Source: CAD feature listing. Evaluate the final solid. Frame: model axes, mm. A direction names the side the tool comes from. Coordinates: 2 decimals unless noted, no trailing zeros. Order: outer loops, then holes, each group sorted by start corner. A loop starts at its lowest first (then second) coordinate and runs counter-clockwise, first axis right, second up. Notation, with made-up numbers: (46, 41.5) -> (69, 41.5) arc R30 ccw to (69, 65.5) -> close; hole circle Ø7 at (4, -16). An arc over 180 degrees is marked (long way). Put each result on its own line as item: value.
from build123d import *

# Parameters (mm, degrees)
CHAMFER3_SIZE = 0.1
CHAMFER4_SIZE = 0.1
CHAMFER5_SIZE = 0.1
CHAMFER6_SIZE = 0.1


with BuildPart() as part:
    # Sketch1 → Revolve2 (revolve)
    with BuildSketch(Plane.XY):
        Polygon((-10.65, 1.5), (0.95, 1.5), (0.95, 0), (22.25, 0), (22.25, -1.5), (0.95, -1.5), (-10.65, -1.5), (-14.75, -1.5), (-14.75, 0), (-10.65, 0), align=None)
    revolve(axis=Axis((-10.65, -1.5, 0), (-1, 0, 0)))

    # Chamfer3
    chamfer3_edges = [part.edges().sort_by_distance(p)[0] for p in [
        (-14.75, -3, 0),
    ]]
    chamfer(chamfer3_edges, length=CHAMFER3_SIZE)

    # Chamfer4
    chamfer4_edges = [part.edges().sort_by_distance(p)[0] for p in [
        (-10.65, -4.5, 0),
    ]]
    chamfer(chamfer4_edges, length=CHAMFER4_SIZE)

    # Chamfer5
    chamfer5_edges = [part.edges().sort_by_distance(p)[0] for p in [
        (0.95, -4.5, 0),
    ]]
    chamfer(chamfer5_edges, length=CHAMFER5_SIZE)

    # Chamfer6
    chamfer6_edges = [part.edges().sort_by_distance(p)[0] for p in [
        (22.25, -3, 0),
    ]]
    chamfer(chamfer6_edges, length=CHAMFER6_SIZE)


solid = part.part
1. Ray query, line 1 along X through (y, z) = (-3, 1.2); line 2 along Y through (x, z) = (18.5, -0.55); line 3 along Z through (x, y) = (-2, -0.75). Return the intervals inside material, ascending.
Numbers:
line 1: x = -10.65 to 0.95
line 2: y = -2.9 to -0.1
line 3: z = -2.9 to 2.9
2. Cut plane B-B on z = 0. Output: boundary loops of the cut face in (x, y).
Numbers:
outline: (-14.75, -2.9) -> (-14.65, -3) -> (-10.65, -3) -> (-10.65, -4.4) -> (-10.55, -4.5) -> (0.85, -4.5) -> (0.95, -4.4) -> (0.95, -3) -> (22.15, -3) -> (22.25, -2.9) -> (22.25, -0.1) -> (22.15, 0) -> (0.95, 0) -> (0.95, 1.4) -> (0.85, 1.5) -> (-10.55, 1.5) -> (-10.65, 1.4) -> (-10.65, 0) -> (-14.65, 0) -> (-14.75, -0.1) -> close
3. Set-up query: faces 1 (the cylindrical face through (-4.8, -3.9, 1.8)), 2 (the cylindrical face through (11.7, -2.7, 0.9)), 3 (the flat face through (-10.65, -3, 1)). Return all of +Z, -Z, +X, -X, +Y, -Y with unobstructed straight access to the full face (end or side cutting, diameter ignored); none if empty.
Numbers:
face 1: +X, -X
face 2: +X
face 3: -X
4. Cut plane A-A on y = -1.5. Output: boundary loops of the cut face in (x, z), plus the area to 3 significant figures.
Numbers:
outline: (-14.75, -1.4) -> (-14.65, -1.5) -> (-10.65, -1.5) -> (-10.65, -2.9) -> (-10.55, -3) -> (0.85, -3) -> (0.95, -2.9) -> (0.95, -1.5) -> (22.15, -1.5) -> (22.25, -1.4) -> (22.25, 1.4) -> (22.15, 1.5) -> (0.95, 1.5) -> (0.95, 2.9) -> (0.85, 3) -> (-10.55, 3) -> (-10.65, 2.9) -> (-10.65, 1.5) -> (-14.65, 1.5) -> (-14.75, 1.4) -> close
area: 146 mm2
5. First-contact query: pin 1 (3 mm diameter, centred on x = 9, y = 0, fed in from +Z); pin 2 (1.5 mm diameter, centred on x = 3, z = -2.5, fed in from -Y); pin 3 (1 mm diameter, centred on x = 0, y = -3.5, fed in from -Z); pin 4 (1 mm diameter, centred on x = -3, z = -2.5, fed in from -Y). Flat tips, straight axial feed; report the tip coordinate or a pass-through.
Numbers:
pin 1: stops at z = 1.5
pin 2: passes through
pin 3: stops at z = -2.6
pin 4: stops at y = -3.74
6. Cut plane D-D on x = -10. Output: boundary loops of the cut face in (y, z).
Numbers:
outline: circle Ø6 at (-1.5, 0)
7. Cut plane C-C on x = 15. Output: boundary loops of the cut face in (y, z), plus the area to 3 significant figures.
Numbers:
outline: circle Ø3 at (-1.5, 0)
area: 7.07 mm2
